from build123d import *

# Parameters (mm, degrees)
F1_DEPTH = 650
F3_DEPTH = 20


with BuildPart() as f1:
    # F0 (on Front) → F1 (new body)
    with BuildSketch(Plane.XZ):
        with BuildLine():
            Line((9, 10), (-9, 10))
            ThreePointArc((-9, 10), (-9.707107, 9.707107), (-10, 9))
            Line((-10, 9), (-10, -9))
            ThreePointArc((-10, -9), (-9.707107, -9.707107), (-9, -10))
            Line((-9, -10), (9, -10))
            ThreePointArc((9, -10), (9.707107, -9.707107), (10, -9))
            Line((10, -9), (10, 9))
            ThreePointArc((10, 9), (9.707107, 9.707107), (9, 10))
        make_face()
        with BuildLine():
            ThreePointArc((-8.75, 7.75), (-8.457107, 8.457107), (-7.75, 8.75))
            Line((-7.75, 8.75), (7.75, 8.75))
            ThreePointArc((7.75, 8.75), (8.457107, 8.457107), (8.75, 7.75))
            Line((8.75, 7.75), (8.75, -7.75))
            ThreePointArc((8.75, -7.75), (8.457107, -8.457107), (7.75, -8.75))
            Line((7.75, -8.75), (-7.75, -8.75))
            ThreePointArc((-7.75, -8.75), (-8.457107, -8.457107), (-8.75, -7.75))
            Line((-8.75, -7.75), (-8.75, 7.75))
        make_face(mode=Mode.SUBTRACT)
    extrude(amount=F1_DEPTH)

    # F2 (on face) → F3 (cut)
    with BuildSketch(Plane.XY.offset(10)):
        Polygon((-9, -650), (9, -650), (9, -649), (-9, -631), align=None)
        Polygon((-10, -650), (-9, -650), (-9, -631), (-10, -630), align=None)
        Polygon((9, -649), (9, -650), (10, -650), align=None)
        Polygon((9, 0), (9, -1), (10, 0), align=None)
        Polygon((-9, -19), (9, -1), (9, 0), (-9, 0), align=None)
        Polygon((-10, -20), (-9, -19), (-9, 0), (-10, 0), align=None)
    extrude(amount=-F3_DEPTH, mode=Mode.SUBTRACT)


solid = f1.part
For this review, take the finished solid that the model builds, in its own axes (mm). A direction names the side the tool comes from. Give positions to 0.01 mm unless a question says otherwise; leave off trailing zeros. Order: outer loops, then holes, each group sorted by start corner. A loop starts at its lowest first (then second) coordinate and runs counter-clockwise, first axis right, second up. Notation, with made-up numbers: (55.5, 64) - (96.5, 64) arc R29 ccw to (96.5, 86) - close; hole circle Ø5 at (18.5, 64.25). An arc over 180 degrees is marked (long way). Answer as a JSON object with one key per item and string values. Group by question number.
Item 1: Take a section at A-A on z = 1. Give the boundary of the cut face in (x, y).
Item 2: Wall thickness on line 1 along X through (y, z) = (-546.5, -6); line 2 along Z through (x, y) = (9.25, -483.5): over which ranges is each line inside the solid? List them lowest first.
Item 3: Machinability: for faces 1 (the flat face through (-8.75, -321, 0)), 2 (the flat face through (0, -10, 9)), which of the approach directions +Z, -Z, +X, -X, +Y, -Y give a long, thin tool a straight path to every point of the face, cutting with its end or side? Answer none if there is none.
Item 4: Clearance check with a flat-ended pin moving along its axis: pin 1 Ø6 at (x, z) = (-5.5, 6.5) entering from -Y. State where the tip first meets the part, or that it passes through.
Item 5: Draft analysis for pull direction X (two halves, no side actions). For faces 3 (the flat face through (8.75, -320, 0)), 4 (the flat face through (0, -320, 10)), 5 (the flat face through (10, -320, 0)), state which applies: pulls with the +X half, pulls with the -X half, needs draft (parallel to the pull), parting line crosses it, or undercut.
Item 6: Take a section at B-B on x = 0.75. Give the boundary of the cut face in (y, z), and give its area (3 significant figures).
Item 7: Take a section at C-C on y = -520.5. Give the boundary of the cut face in (x, z), and give its area (4 significant figures).
Reported:
{
 "1": {"outline": "(-10, -630) - (-8.75, -631.25) - (-8.75, -18.75) - (-10, -20) - close; (8.75, -648.75) - (10, -650) - (10, 0) - (8.75, -1.25) - close"},
 "2": {"line 1": "-10 to -8.75, 8.75 to 10", "line 2": "-9.97 to 9.97"},
 "3": {"face 1": "+Y, -Y", "face 2": "+Z, -Z, -X, +Y"},
 "4": {"pin 1": "y = -636.48"},
 "5": {"face 3": "undercut", "face 4": "needs draft", "face 5": "pulls with the +X half"},
 "6": {"outline": "(-640.75, -10) - (-9.25, -10) - (-9.25, -8.75) - (-640.75, -8.75) - close; (-640.75, 8.75) - (-9.25, 8.75) - (-9.25, 10) - (-640.75, 10) - close", "area": "1,580 mm^2"},
 "7": {"outline": "(-10, -9) arc R1 ccw to (-9, -10) - (9, -10) arc R1 ccw to (10, -9) - (10, 9) arc R1 ccw to (9, 10) - (-9, 10) arc R1 ccw to (-10, 9) - close; hole (-8.75, -7.75) arc R1 ccw to (-7.75, -8.75) - (7.75, -8.75) arc R1 ccw to (8.75, -7.75) - (8.75, 7.75) arc R1 ccw to (7.75, 8.75) - (-7.75, 8.75) arc R1 ccw to (-8.75, 7.75) - close", "area": "93.75 mm^2"}
}
